```python
from build123d import *

# Parameters (mm, degrees)
SKETCH_1_R          = 7.1
EXTRUDE_1_DEPTH     = 8
SKETCH_2_R          = 1.7
CUT_EXTRUDE_1_DEPTH = 6
SKETCH_3_R          = 5.1
CUT_EXTRUDE_2_DEPTH = 5
SKETCH_4_R          = 3.7
SKETCH_4_R_2        = 1.7
EXTRUDE_2_DEPTH     = 8
CUT_EXTRUDE_4_DEPTH = 5


with BuildPart() as part:
    # 草图1 → 凸台-拉伸1 (new body)
    with BuildSketch(Plane.XY):
        with Locations((-2.763223282, 3.564558034)):
            Circle(SKETCH_1_R)
    extrude(amount=EXTRUDE_1_DEPTH)

    # 草图2 → 切除-拉伸1 (cut)
    with BuildSketch(Plane(origin=(0, 0, 0), x_dir=(-1, 0, 0), z_dir=(0, 0, -1))):
        with Locations((2.763223282, 3.564558034)):
            Circle(SKETCH_2_R)
    extrude(amount=-CUT_EXTRUDE_1_DEPTH, mode=Mode.SUBTRACT)

    # 草图3 → 切除-拉伸2 (cut)
    with BuildSketch(Plane.XY.offset(8)):
        with Locations((-2.763223282, 3.564558034)):
            Circle(SKETCH_3_R)
    extrude(amount=-CUT_EXTRUDE_2_DEPTH, mode=Mode.SUBTRACT)

    # 草图4 → 凸台-拉伸2 (add)
    with BuildSketch(Plane(origin=(0, 0, 0), x_dir=(-1, 0, 0), z_dir=(0, 0, -1))):
        with Locations((2.763223282, 3.564558034)):
            Circle(SKETCH_4_R)
        with Locations((2.763223282, 3.564558034)):
            Circle(SKETCH_4_R_2, mode=Mode.SUBTRACT)
    extrude(amount=EXTRUDE_2_DEPTH)

    # 草图5 → 切除-拉伸4 (cut)
    with BuildSketch(Plane.XY.offset(8)):
        with BuildLine():
            Line((-0.763223282, 4.719258572), (-0.763223282, 10.377046566))
            ThreePointArc((-0.763223282, 10.377046566), (-2.763223282, 10.664558034), (-4.763223282, 10.377046566))
            Line((-4.763223282, 10.377046566), (-4.763223282, 4.719258572))
            Line((-4.763223282, 4.719258572), (-9.663011414, 1.890364575))
            ThreePointArc((-9.663011414, 1.890364575), (-8.912003649, 0.014558034), (-7.663011414, -1.57373704))
            Line((-7.663011414, -1.57373704), (-2.763223282, 1.255156957))
            Line((-2.763223282, 1.255156957), (2.13656485, -1.57373704))
            ThreePointArc((2.13656485, -1.57373704), (3.385557085, 0.014558034), (4.13656485, 1.890364575))
            Line((4.13656485, 1.890364575), (-0.763223282, 4.719258572))
        make_face()
    extrude(amount=-CUT_EXTRUDE_4_DEPTH, mode=Mode.SUBTRACT)


solid = part.part
```
The listing builds one solid part. Answer for the finished solid, in the listing's coordinates (mm). A direction names the side the tool comes from. Give positions to 0.01 mm unless a question says otherwise; leave off trailing zeros. Order: outer loops, then holes, each group sorted by start corner. A loop starts at its lowest first (then second) coordinate and runs counter-clockwise, first axis right, second up. Notation, with made-up numbers: (-27.5, 59) - (-18.5, 59) arc R19 ccw to (-18.5, 85) - close; hole circle Ø5 at (89.5, 84). An arc over 180 degrees is marked (long way). Answer in a Markdown table with one row per item. Add a question column.
Q1. Given P1, Ø3, axis at x = -8.5, z = 0, coming from the -Y side; P2, Ø2.5, axis at y = 9.5, z = 6, coming from the +X side; P3, Ø4, axis at x = 1.5, y = -0.5, coming from the +Z side; P4, Ø0.8, axis at x = -3, y = -0.5, coming from the +Z side, each flat-ended and moving along its own axis, determine where each tip first touches the part or whether it passes through.
Q2. The part is cut by section D-D (x = 0). Determine the outline of the cut face in (y, z).
Q3. The part is cut by section C-C (y = 9.5). Determine the outline of the cut face in (x, z).
Q4. Which of the six approach directions +Z, -Z, +X, -X, +Y, -Y give full straight-line access (tool end or side, diameter ignored) to faces 1 (the cylindrical face through (-7.16, 6.15, 5.54)), 2 (the flat face through (-6.757, -1.051, 5.535)), 3 (the flat face through (-0.763, 9, 6)), 4 (the flat face through (0.3, 0.5, 0))?
Q5. The part is cut by section A-A (z = 6.5). Determine the outline of the cut face in (x, y).
Q6. For a pull along Y with two mould halves and no side action, classify faces 5 (the flat face through (-4.763, 9, 6)), 6 (the cylindrical face through (-0.04, 6.07, -3.94)), 7 (the flat face through (1.21, -1.04, 5.54)) as released by +Y, released by -Y, zero draft, split by the parting line, or undercut.
Q7. Find the intervals of material crossed by line 1 along Z through (x, y) = (-2.75, 6.5); line 2 along Z through (x, y) = (-8, 2); line 3 along X through (y, z) = (3.5, -3.75), in increasing order. Write a range as [from, to].
Q8. The part is cut by section B-B (x = -3.25). Determine the outline of the cut face in (y, z).
Determined:
| question | item | result |
|---|---|---|
| 1 | P1 | stops at y = -2.13 |
| 1 | P2 | stops at x = 2.57 |
| 1 | P3 | stops at z = 8 |
| 1 | P4 | stops at z = 3 |
| 2 | outline | (-2.98, 0) - (1.1, 0) - (1.1, -8) - (6.03, -8) - (6.03, 0) - (10.1, 0) - (10.1, 8) - (7.85, 8) - (7.85, 3) - (-0.72, 3) - (-0.72, 8) - (-2.98, 8) - close |
| 3 | outline | (-6.66, 0) - (1.13, 0) - (1.13, 8) - (-0.76, 8) - (-0.76, 3) - (-4.76, 3) - (-4.76, 8) - (-6.66, 8) - close |
| 4 | face 1 | +Z |
| 4 | face 2 | +Z, -X |
| 4 | face 3 | +Z, +Y |
| 4 | face 4 | -Z |
| 5 | outline | (-9.66, 1.89) - (-7.83, 2.95) arc R5.1 cw to (-4.76, 8.26) - (-4.76, 10.38) arc R7.1 ccw to start; (-7.66, -1.57) arc R7.1 ccw to (2.14, -1.57) - (0.3, -0.51) arc R5.1 cw to (-5.83, -0.51) - close; (-0.76, 8.26) arc R5.1 cw to (2.3, 2.95) - (4.14, 1.89) arc R7.1 ccw to (-0.76, 10.38) - close |
| 6 | face 5 | zero draft |
| 6 | face 6 | split by the parting line |
| 6 | face 7 | undercut |
| 7 | line 1 | z = [-8, 3] |
| 7 | line 2 | z = [0, 3] |
| 7 | line 3 | x = [-6.46, -4.46], [-1.06, 0.94] |
| 8 | outline | (-3.52, 0) - (-0.1, 0) - (-0.1, -8) - (1.94, -8) - (1.94, 3) - (-1.51, 3) - (-1.51, 8) - (-3.52, 8) - close; (5.19, -8) - (7.23, -8) - (7.23, 0) - (10.65, 0) - (10.65, 3) - (5.19, 3) - close |
